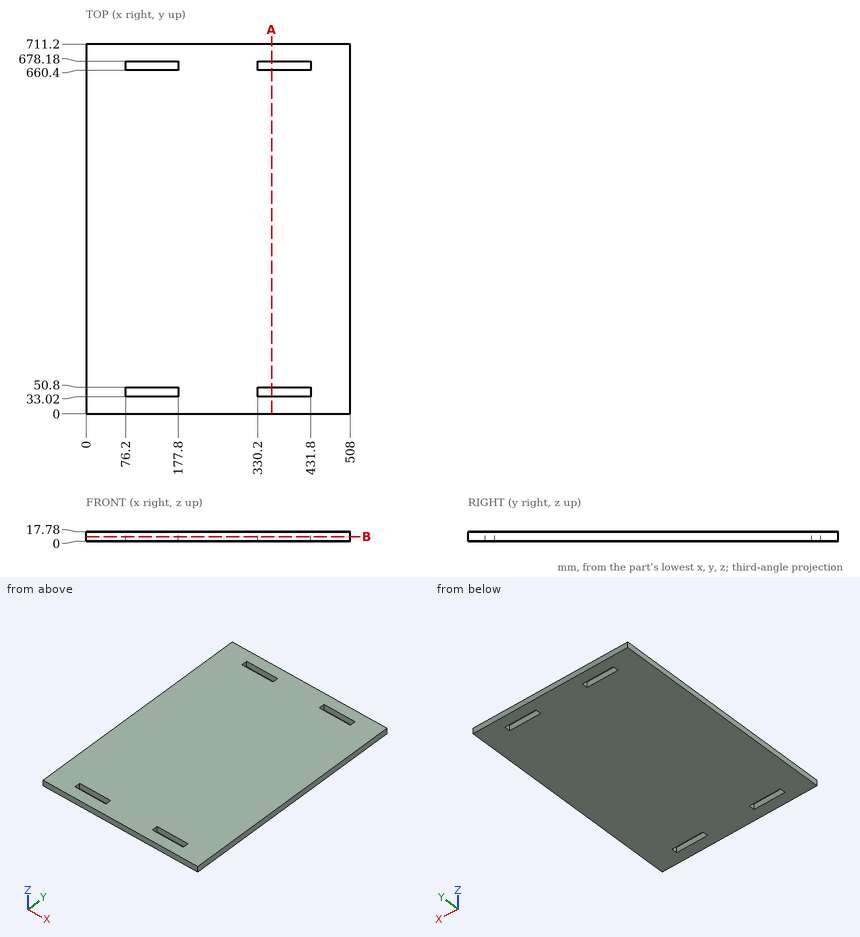
Input: dimensioned drawing with shaded views. Units: mm. Origin: part minimum x, y, z. Round coordinates to 2 decimals unless told otherwise and drop trailing zeros. Loops run counter-clockwise (first coordinate to the right, second up) from the corner with the lowest first, then second, coordinate; pieces in that order, holes last. Notation, with made-up numbers: M -22.75,87 L -9.75,87 A19 ccw -9.75,97 Z; hole C 2.25,3 d6. An arc over 180 degrees is marked long. Answer in a Markdown table with one row per item. Add a question column.
1. Ray query, probe 1 along Y at (x, z) = (158.5, 1.5). Return the intervals inside material, ascending.
2. Section A-A (x = 357). Output: boundary loops of the cut face in (y, z), and give its area (3 significant figures).
3. Section B-B (z = 8.5). Output: boundary loops of the cut face in (x, y), and give its area (3 significant figures).
Values follow:
| question | item | result |
|---|---|---|
| 1 | probe 1 | 0 to 33.02, 50.8 to 660.4, 678.18 to 711.2 |
| 2 | outline | M 0,0 L 33.02,0 L 33.02,17.78 L 0,17.78 Z; M 50.8,0 L 660.4,0 L 660.4,17.78 L 50.8,17.78 Z; M 678.18,0 L 711.2,0 L 711.2,17.78 L 678.18,17.78 Z |
| 2 | area | 12,000 mm^2 |
| 3 | outline | M 0,0 L 508,0 L 508,711.2 L 0,711.2 Z; hole M 76.2,33.02 L 177.8,33.02 L 177.8,50.8 L 76.2,50.8 Z; hole M 76.2,660.4 L 177.8,660.4 L 177.8,678.18 L 76.2,678.18 Z; hole M 330.2,33.02 L 431.8,33.02 L 431.8,50.8 L 330.2,50.8 Z; hole M 330.2,660.4 L 431.8,660.4 L 431.8,678.18 L 330.2,678.18 Z |
| 3 | area | 354,000 mm^2 |
